Work out the finished part from the listing and answer in its coordinate system (mm). A direction names the side the tool comes from. Coordinates: 2 decimals unless noted, no trailing zeros. Order: outer loops, then holes, each group sorted by start corner. A loop starts at its lowest first (then second) coordinate and runs counter-clockwise, first axis right, second up. Notation, with made-up numbers: (55, -25.5) -> (82, -25.5) arc R8 ccw to (82, -11.5) -> close; hole circle Ø5 at (45.5, 74.25). An arc over 180 degrees is marked (long way). Use one line per item in the form item = value.
Autodesk Inventor part; units mm, degrees
ref_plane "YZ Plane" through (0, 0, 0) normal (1, 0, 0) x (0, 1, 0)
ref_plane "XZ Plane" through (0, 0, 0) normal (0, 1, 0) x (-1, 0, 0)
ref_plane "XY Plane" through (0, 0, 0) normal (0, 0, 1) x (1, 0, 0)
sketch "スケッチ1" plane through (0, 0, 0) normal (0, 1, 0) x (-1, 0, 0)
  circle A0 centre (0, 0) radius 86.2565
  circle A1 centre (0, 0) radius 6.25
  dimension "d0" = 172.513
  dimension "d1" = 12.5
extrude "押し出し1" add sketch "スケッチ1" along normal blind 3
sketch "スケッチ2" plane through (0, 3, 0) normal (0, 1, 0) x (1, 0, 0)
  circle A0 centre (0, 0) radius 50.75
  point P0 (0, 50.75)
  point P1 (-50.75, 0)
  point P2 (0, -50.75)
  point P3 (50.75, 0)
  dimension "d4" = 101.5
  dimension "d7" = 360
hole "穴1" at (0, 3, -50.75) at (-50.75, 3, 0) at (0, 3, 50.75) at (50.75, 3, 0) direction (0, -1, 0) diameter 4.3 end through all
sketch "スケッチ3" plane through (0, 3, 0) normal (0, 1, 0) x (1, 0, 0)
  line L0 (0, 0) -> (86.2565, 0)
  circle A0 centre (0, 0) radius 86.2565
  circle A1 centre (0, 0) radius 6.25
  line L1 (0, 0) -> (60.9926, -60.9926)
  line L2 (1.0606, -86.25) -> (-86.25, 1.0606)
  line L3 (86.25, -1.0606) -> (-1.0606, 86.25)
  point P0 (-1.0606, 86.25)
  point P1 (85.1894, 0)
  point P2 (86.25, -1.0606)
  dimension "d16" = 45
  dimension "d17" = 60.238
extrude "押し出し2" cut sketch "スケッチ3" against normal blind 3 contours L3 A0 L0 | L0 A0 L3 | A0 L2
sketch "スケッチ4" plane through (0, 3, 0) normal (0, 1, 0) x (1, 0, 0)
  circle A0 centre (0, 0) radius 6.25
  circle A1 centre (0, 0) radius 12
  line L0 (0, 0) -> (-8.4853, -8.4853)
  line L1 (0, 0) -> (-12, 0)
  point P0 (3.1058, -11.5911)
  point P1 (11.5911, -3.1058)
  point P2 (8.4853, 8.4853)
  point P3 (-3.1058, 11.5911)
  point P4 (-11.5911, 3.1058)
  dimension "d20" = 24
  dimension "d21" = 45
  dimension "d24" = 360
hole "穴2" at (-8.4853, 3, 8.4853) at (3.1058, 3, 11.5911) at (11.5911, 3, 3.1058) at (8.4853, 3, -8.4853) at (-3.1058, 3, -11.5911) at (-11.5911, 3, -3.1058) direction (0, -1, 0) diameter 4.3 end through all
sketch "スケッチ5" plane through (0, 3, 0) normal (0, 1, 0) x (1, 0, 0)
  arc A0 (1.0606, -86.25) -> (86.25, -1.0606) centre (0, 0) ccw
  line L0 (14.0562, -85.1035) -> (-85.1035, 14.0562)
  arc A1 (-1.0606, 86.25) -> (-86.25, 1.0606) centre (0, 0) ccw
  line L1 (-86.25, 1.0606) -> (1.0606, -86.25)
  line L2 (-14.0562, 85.1035) -> (85.1035, -14.0562)
  line L3 (86.25, -1.0606) -> (-1.0606, 86.25)
  line L4 (-86.25, 1.0606) -> (-1.0606, 86.25)
  line L5 (1.0606, -86.25) -> (86.25, -1.0606)
  line L6 (-73.8926, 2.8453) -> (-2.8453, 73.8926)
  line L7 (80.9636, 4.2257) -> (2.8453, -73.8926)
  point P0 (73.8926, -2.8453)
  dimension "d33" = 10
  dimension "d34" = 10
  dimension "d35" = 7.476
  dimension "d36" = 7.476
hole "穴3" at (-73.8926, 3, -2.8453) at (-2.8453, 3, -73.8926) at (73.8926, 3, 2.8453) at (2.8453, 3, 73.8926) direction (0, -1, 0) diameter 3.2 end through all
sketch "スケッチ6" plane through (0, 3, 0) normal (0, 1, 0) x (1, 0, 0)
  circle A0 centre (0, 0) radius 6.25
  circle A1 centre (0, 0) radius 70
  circle A2 centre (0, 0) radius 50
  circle A3 centre (-2.8453, 73.8926) radius 1.6
  line L0 (0, 0) -> (-2.8453, 73.8926)
  circle A4 centre (-73.8926, 2.8453) radius 1.6
  line L1 (0, 0) -> (-73.8926, 2.8453)
  line L2 (0, 0) -> (-20.7056, 66.8676)
  line L3 (0, 0) -> (-66.8676, 20.7056)
  circle A5 centre (0, 0) radius 25
  circle A6 centre (0, 50.75) radius 2.15
  line L4 (0, 0) -> (0, 50.75)
  line L5 (0, 0) -> (8.6824, 49.2404)
  line L6 (0, 0) -> (49.2404, 8.6824)
  circle A7 centre (50.75, 0) radius 2.15
  line L7 (0, 0) -> (50.75, 0)
  line L8 (0, 0) -> (-49.2404, -8.6824)
  line L9 (0, 0) -> (-8.6824, -49.2404)
  line L10 (0, 0) -> (20.7056, -66.8676)
  line L11 (0, 0) -> (66.8676, -20.7056)
  circle A8 centre (0, 0) radius 40
  point P0 (-4.3412, -24.6202)
  point P1 (-24.6202, -4.3412)
  point P2 (47.7626, -14.7897)
  point P3 (23.8813, -7.3948)
  point P4 (7.3948, -23.8813)
  point P5 (14.7897, -47.7626)
  point P6 (24.6202, 4.3412)
  point P7 (4.3412, 24.6202)
  point P8 (-23.8813, 7.3948)
  point P9 (-7.3948, 23.8813)
  point P10 (-14.7897, 47.7626)
  point P11 (-47.7626, 14.7897)
  point P12 (66.8676, -20.7056)
  point P13 (20.7056, -66.8676)
  point P14 (38.2101, -11.8318)
  point P15 (11.8318, -38.2101)
  point P16 (-38.2101, 11.8318)
  point P17 (-11.8318, 38.2101)
  dimension "d44" = 140
  dimension "d45" = 100
  dimension "d46" = 15
  dimension "d47" = 15
  dimension "d48" = 50
  dimension "d49" = 10
  dimension "d50" = 10
  dimension "d53" = 360
  dimension "d57" = 80
extrude "押し出し3" cut sketch "スケッチ6" against normal blind 10 contours A5 L5 A8 L6 | L11 A8 L10 A5 | A8 L5 A2 L6 | L11 A2 L10 A8 | A5 L3 A8 L2 | A5 L9 A8 L8 | L11 A1 L10 A2 | A8 L3 A2 L2 | A8 L9 A2 L8 | A2 L3 A1 L2
fillet "フィレット1" radius 5 14 edges at (-20.7056, 1.5, -66.8676) (-66.8676, 1.5, -20.7056) (-49.2404, 1.5, 8.6824) (-24.6202, 1.5, 4.3412) (-8.6824, 1.5, 49.2404) (-4.3412, 1.5, 24.6202) (20.7056, 1.5, 66.8676) (66.8676, 1.5, 20.7056) (24.6202, 1.5, -4.3412) (49.2404, 1.5, -8.6824) (8.6824, 1.5, -49.2404) (4.3412, 1.5, -24.6202) (-7.3948, 1.5, -23.8813) (-23.8813, 1.5, -7.3948)
properties part number "baseplate_R2toR3" material "アルミニウム 6061"
(1) Section C-C on y = 0.45 is taken. Count the separate pieces of the cut face and the enclosed holes in it, plus the area to 3 significant figures.
Data:
separate_pieces = 1
enclosed_holes = 19
area = 12,300 mm²
(2) The mould has two halves that part along Z. Classify faces 1 (the cylindrical face through (-61.65, 1.48, -60.33)), 2 (the flat face through (-41.98, 1.52, 43.21)), 3 (the cylindrical face through (47.45, 1.48, -10.1)): released by +Z, released by -Z, zero draft, split by the parting line, or undercut.
Data:
face_1 = released by -Z
face_2 = released by +Z
face_3 = undercut
(3) Section B-B on z = 50.75 is taken. Write down the section's boundary in (x, y), plus the area to 3 significant figures.
Data:
outline = (-34.44, 0) -> (-2.15, 0) -> (-2.15, 3) -> (-34.44, 3) -> close; (2.15, 0) -> (15.71, 0) -> (15.71, 3) -> (2.15, 3) -> close; (48.21, 0) -> (69.75, 0) -> (69.75, 3) -> (48.21, 3) -> close
area = 202 mm²
(4) Which of the six approach directions +Z, -Z, +X, -X, +Y, -Y give full straight-line access (tool end or side, diameter ignored) to faces 4 (the cylindrical face through (61.65, 1.48, 60.33)), 5 (the cylindrical face through (35.6, 1.52, -35.11))?
Data:
face_4 = +Z, +X, +Y, -Y
face_5 = +Y, -Y
(5) Straight lines are drawn through the part: line 1 along Z through (x, y) = (39, 2.3); line 2 along X through (y, z) = (0.6, -20); line 3 along X through (y, z) = (1.15, 45). For each, find the intervals that lie inside material, in ascending order.
Data:
line_1 = -46.19 to -31.29, -6.88 to 12.08, 58.13 to 76.94
line_2 = -83.91 to -63.5, -15 to 15, 45.83 to 65.19
line_3 = -40.19 to -21.79, -8.04 to 13.93, 53.62 to 73.59
(6) Each of these flat-tipped pins is pushed along its axis until it touches: P1, Ø3, axis at x = -73.89, z = -2.85, coming from the -Y side; P2, Ø1, axis at y = 2, z = 1.5, coming from the -X side. Where does it stop, or does it pass through?
Data:
P1 = through
P2 = -84.19
(7) Section A-A on x = -35 is taken. Write down the section's boundary in (y, z), plus the area to 3 significant figures.
Data:
outline = (0, -78.84) -> (3, -78.84) -> (3, -60.62) -> (0, -60.62) -> close; (0, -10.84) -> (3, -10.84) -> (3, 6.17) -> (0, 6.17) -> close; (0, 35.71) -> (3, 35.71) -> (3, 50.19) -> (0, 50.19) -> close
area = 149 mm²
